Can you work these out from the model? Positions are in its coordinate system, mm. A direction names the side the tool comes from. Round coordinates to 2 decimals unless told otherwise and drop trailing zeros. Loops run counter-clockwise (first coordinate to the right, second up) from the corner with the lowest first, then second, coordinate; pieces in that order, holes last. Notation, with made-up numbers: (-15.75, -26.5) - (-9.75, -26.5) arc R10 cw to (-9.75, -13.5) - close; hole circle Ø5 at (74.5, 76.25). An arc over 180 degrees is marked (long way). Answer as CSV lines item,"result".
```python
from build123d import *

# Parameters (mm, degrees)
SKETCH1_W           = 35
SKETCH1_H           = 50
BOSS_EXTRUDE1_DEPTH = 10
SKETCH2_W           = 35
SKETCH2_H           = 10
BOSS_EXTRUDE2_DEPTH = 40
SKETCH3_R           = 2
CUT_EXTRUDE1_DEPTH  = 30
SKETCH4_R           = 2
CUT_EXTRUDE2_DEPTH  = 30
BOSS_EXTRUDE3_DEPTH = 35
SKETCH6_R           = 3.5
CUT_EXTRUDE3_DEPTH  = 30
SKETCH7_R           = 3.5
CUT_EXTRUDE4_DEPTH  = 30


with BuildPart() as part:
    # Sketch1 → Boss-Extrude1 (new body)
    with BuildSketch(Plane.XY):
        with Locations((-5.304878049, 18.567073171)):
            Rectangle(SKETCH1_W, SKETCH1_H)
    extrude(amount=BOSS_EXTRUDE1_DEPTH)

    # Sketch2 → Boss-Extrude2 (add)
    with BuildSketch(Plane.XY.offset(10)):
        with Locations((-5.304878049, 38.567073171)):
            Rectangle(SKETCH2_W, SKETCH2_H)
    extrude(amount=BOSS_EXTRUDE2_DEPTH)

    # Sketch3 → Cut-Extrude1 (cut)
    with BuildSketch(Plane.XY.offset(10)):
        with Locations((5.195121951, 0.567073171)):
            Circle(SKETCH3_R)
        with Locations((-15.804878049, 18.567073171)):
            Circle(SKETCH3_R)
        with Locations((5.195121951, 18.567073171)):
            Circle(SKETCH3_R)
        with Locations((-15.804878049, 0.567073171)):
            Circle(SKETCH3_R)
    extrude(amount=-CUT_EXTRUDE1_DEPTH, mode=Mode.SUBTRACT)

    # Sketch4 → Cut-Extrude2 (cut)
    with BuildSketch(Plane.XZ.offset(-33.567073171)):
        with Locations(Location((-15.804878049, 43, 0), (0, 0, 270))):
            Circle(SKETCH4_R)
        with Locations(Location((5.195121951, 43, 0), (0, 0, 270))):
            Circle(SKETCH4_R)
        with Locations(Location((-15.804878049, 25, 0), (0, 0, 270))):
            Circle(SKETCH4_R)
        with Locations(Location((5.195121951, 25, 0), (0, 0, 270))):
            Circle(SKETCH4_R)
    extrude(amount=-CUT_EXTRUDE2_DEPTH, mode=Mode.SUBTRACT)

    # Sketch5 → Boss-Extrude3 (add)
    with BuildSketch(Plane.ZY.offset(22.804878049)):
        Polygon((30, 33.567073171), (10, 13.567073171), (10, 33.567073171), align=None)
    extrude(amount=-BOSS_EXTRUDE3_DEPTH)

    # Sketch6 → Cut-Extrude3 (cut)
    with BuildSketch(Plane(origin=(0, 33.567073171, 0), x_dir=(1, 0, 0), z_dir=(0, 1, 0))):
        with Locations(Location((5.195121951, -25, 0), (0, 0, 180))):
            Circle(SKETCH6_R)
        with Locations(Location((-15.804878049, -25, 0), (0, 0, 180))):
            Circle(SKETCH6_R)
    extrude(amount=-CUT_EXTRUDE3_DEPTH, mode=Mode.SUBTRACT)

    # Sketch7 → Cut-Extrude4 (cut)
    with BuildSketch(Plane(origin=(0, 0, 10), x_dir=(-1, 0, 0), z_dir=(0, 0, -1))):
        with Locations((-5.195121951, 18.567073171)):
            Circle(SKETCH7_R)
        with Locations((15.804878049, 18.567073171)):
            Circle(SKETCH7_R)
    extrude(amount=-CUT_EXTRUDE4_DEPTH, mode=Mode.SUBTRACT)


solid = part.part
```
Q1. Imagine slicing it at D-D (z = 4). Write out the boundary of the cut face in (x, y), then the cut area to 3 significant figures.
Checks:
outline,"(-22.8, -6.43) - (12.2, -6.43) - (12.2, 43.57) - (-22.8, 43.57) - close; hole circle Ø4 at (-15.8, 0.57); hole circle Ø4 at (-15.8, 18.57); hole circle Ø4 at (5.2, 0.57); hole circle Ø4 at (5.2, 18.57)"
area,"1,700 mm²"
Q2. I'm going to push flat-ended pins straight in: pin 1 Ø3.5 at (x, y) = (-14.5, 20) entering from +Z; pin 2 Ø5.5 at (x, z) = (5, 24) entering from -Y; pin 3 Ø8 at (x, y) = (-10, 11) entering from +Z; pin 4 Ø3.5 at (x, y) = (5.2, 18.57) entering from +Z. Where does each tip first touch, or does it pass through?
Checks:
pin 1,"z = 18.17"
pin 2,"y = 24.82"
pin 3,"z = 11.43"
pin 4,"through"
Q3. Imagine slicing it at B-B (x = -4). Write out the boundary of the cut face in (y, z).
Checks:
outline,"(-6.43, 0) - (43.57, 0) - (43.57, 50) - (33.57, 50) - (33.57, 30) - (13.57, 10) - (-6.43, 10) - close"
Q4. Imagine slicing it at A-A (z = 43). Write out the boundary of the cut face in (x, y), then the cut area to 3 significant figures.
Checks:
outline,"(-22.8, 33.57) - (-17.8, 33.57) - (-17.8, 43.57) - (-22.8, 43.57) - close; (-13.8, 33.57) - (3.2, 33.57) - (3.2, 43.57) - (-13.8, 43.57) - close; (7.2, 33.57) - (12.2, 33.57) - (12.2, 43.57) - (7.2, 43.57) - close"
area,"270 mm²"
Q5. On a 3-axis mill with a long thin cutter (end or side, diameter ignored), from which of +Z, -Z, +X, -X, +Y, -Y can I reach the whole of each face in a straight line? I mean faces 5 (the flat face through (4, 33.567, 23)), 6 (the flat face through (-6, 4, 10)), 7 (the cylindrical face through (-17.8, 0.7, 5.1)), 8 (the flat face through (-6, -6.433, 5)), 9 (the flat face through (-16, 16, 10)). Say none if no direction works.
Checks:
face 5,"-Y"
face 6,"+Z, +X, -X, -Y"
face 7,"+Z, -Z"
face 8,"+Z, -Z, +X, -X, -Y"
face 9,"+Z"
Q6. We'd pull the mould along Z, two halves only. Please class faces 1 (the flat face through (-22.805, 30, 14)), 2 (the cylindrical face through (-15.046, 30.289, 21.583)), 3 (the flat face through (3, 19, 10)), 4 (the cylindrical face through (-17.76, 38.5, 25.43)): pulls with the +Z half, pulls with the -Z half, needs draft (parallel to the pull), parting line crosses it, or undercut.
Checks:
face 1,"needs draft"
face 2,"undercut"
face 3,"pulls with the +Z half"
face 4,"undercut"
Q7. If I drill on line 1 along X through (y, z) = (38.25, 25); line 2 along Z through (x, y) = (5.5, 41.5); line 3 along Z through (x, y) = (7, 40.5), over which ranges is the centre line in solid material (lowest first)? Write a range as [from, to].
Checks:
line 1,"[-22.8, -17.8], [-13.8, 3.2], [7.2, 12.2]"
line 2,"[0, 23.02], [26.98, 41.02], [44.98, 50]"
line 3,"[0, 24.14], [25.86, 42.14], [43.86, 50]"
Q8. Imagine slicing it at C-C (y = 39). Write out the boundary of the cut face in (x, z), then the cut area to 3 significant figures.
Checks:
outline,"(-22.8, 0) - (12.2, 0) - (12.2, 50) - (-22.8, 50) - close; hole circle Ø4 at (-15.8, 25); hole circle Ø4 at (-15.8, 43); hole circle Ø4 at (5.2, 25); hole circle Ø4 at (5.2, 43)"
area,"1,700 mm²"
